Here's how the part is built. I have some questions about the finished solid (model axes, mm). A direction names the side the tool comes from. Coordinates: 2 decimals unless noted, no trailing zeros. Write each loop counter-clockwise with the first axis right and the second up, starting at its lowest first coordinate (ties: lowest second). Pieces come first, ordered by that corner, then holes.
(1) Imagine slicing it at C-C, the plane y = -25.5. List the corners of the cut face in (x, z) for me, plus the area to 3 significant figures.
(2) Which directions (+Z, -Z, +X, -X, +Y, -Y) give clear straight access to the entire face, cutting with the end or side of a thin tool? Please do faces 4 (the flat face through (23.3, -114.3, 10.6)), 5 (the flat face through (1, 0, 27)).
(3) For pin 1 Ø10 at (y, z) = (-74.5, 4) entering from -X; pin 2 Ø1 at (x, z) = (39, 24) entering from +Y; pin 3 Ø6 at (x, z) = (34, 19.5) entering from -Y; pin 4 Ø12 at (y, z) = (-80, -30) entering from -X, each with a flat end and sliding along its axis, tell me the tip position at first contact or that it passes through.
(4) Thinking about a two-plate mould opening in Y: for faces 1 (the flat face through (0, -177.8, 0)), 2 (the cylindrical face through (15.259, -56.35, 48.454)), 3 (the cylindrical face through (-0.83, -22.37, 0.18)), which applies, released by +Y, released by -Y, zero draft, split by the parting line, or undercut?
(5) Imagine slicing it at A-A, the plane x = 0. List the corners of the cut face in (y, z) for me.
(6) Imagine slicing it at D-D, the plane x = -38. List the corners of the cut face in (y, z) for me.
(7) Imagine slicing it at B-B, the plane z = 0. List the corners of the cut face in (x, y) for me.
(8) Please list where these lines run through material, in increasing order: probe 1 along Y at (x, z) = (-8, -27); probe 2 along Z at (x, y) = (-45, -11.5); probe 3 along Y at (x, z) = (-46, 3.5).
```python
from build123d import *

# Parameters (mm, degrees)
SKETCH1_R           = 50.8
BOSS_EXTRUDE1_DEPTH = 114.3
SKETCH2_R           = 25.4
BOSS_EXTRUDE2_DEPTH = 63.5
SKETCH3_W           = 130.646832002
SKETCH3_H           = 25.4
CUT_EXTRUDE5_DEPTH  = 50.8
SKETCH5_R           = 6.35
BOSS_EXTRUDE3_DEPTH = 50.8


with BuildPart() as part:
    # Sketch1 → Boss-Extrude1 (new body)
    with BuildSketch(Plane(origin=(0, 0, 0), x_dir=(1, 0, 0), z_dir=(0, 1, 0))):
        with Locations(Location((0, 0, 0), (0, 0, 270))):
            Circle(SKETCH1_R)
    extrude(amount=-BOSS_EXTRUDE1_DEPTH)

    # Sketch2 → Boss-Extrude2 (add)
    with BuildSketch(Plane(origin=(0, -114.3, 0), x_dir=(-1, 0, 0), z_dir=(0, -1, 0))):
        with Locations(Location((0, 0, 0), (0, 0, 90))):
            Circle(SKETCH2_R)
    extrude(amount=BOSS_EXTRUDE2_DEPTH)

    # Sketch3 → Cut-Extrude5 (cut)
    with BuildSketch(Plane(origin=(0, 0, 0), x_dir=(1, 0, 0), z_dir=(0, 1, 0))):
        Rectangle(SKETCH3_W, SKETCH3_H)
    extrude(amount=-CUT_EXTRUDE5_DEPTH, mode=Mode.SUBTRACT)

    # Sketch5 → Boss-Extrude3 (add)
    with BuildSketch(Plane(origin=(0, 0, 12.7), x_dir=(-1, 0, 0), z_dir=(0, 0, -1))):
        with Locations(Location((0, -16.075927957, 0), (0, 0, 180))):
            Circle(SKETCH5_R)
    extrude(amount=BOSS_EXTRUDE3_DEPTH)


solid = part.part
```
Recorded:
1. outline: (-49.19, -12.7) arc R50.8 ccw to (49.19, -12.7) - close; (-49.19, 12.7) - (49.19, 12.7) arc R50.8 ccw to start
1. area: 5,550 mm2
2. face 4: -Y
2. face 5: +Z, -Z, +X, -X, +Y
3. pin 1: stops at x = -50.8
3. pin 2: stops at y = 0
3. pin 3: stops at y = -114.3
3. pin 4: stops at x = -44.77
4. face 1: released by -Y
4. face 2: zero draft
4. face 3: undercut
5. outline: (-177.8, -25.4) - (-114.3, -25.4) - (-114.3, -50.8) - (0, -50.8) - (0, -12.7) - (-9.73, -12.7) - (-9.73, 12.7) - (0, 12.7) - (0, 50.8) - (-114.3, 50.8) - (-114.3, 25.4) - (-177.8, 25.4) - close; hole (-50.8, -12.7) - (-22.43, -12.7) - (-22.43, 12.7) - (-50.8, 12.7) - close
6. outline: (-114.3, -33.71) - (0, -33.71) - (0, -12.7) - (-50.8, -12.7) - (-50.8, 12.7) - (0, 12.7) - (0, 33.71) - (-114.3, 33.71) - close
7. outline: (-50.8, -114.3) - (-25.4, -114.3) - (-25.4, -177.8) - (25.4, -177.8) - (25.4, -114.3) - (50.8, -114.3) - (50.8, -50.8) - (-50.8, -50.8) - close; circle Ø12.7 at (0, -16.08)
8. probe 1: y = -114.3 to 0
8. probe 2: z = -23.57 to -12.7, 12.7 to 23.57
8. probe 3: y = -114.3 to -50.8
